```python
from build123d import *

# Parameters (mm, degrees)
F0_R     = 7
F1_DEPTH = 25


with BuildPart() as f1:
    # F0 (on Top) → F1 (new body)
    with BuildSketch(Plane.XY):
        with BuildLine():
            Line((-14, 10.835116), (-14, -7.164884))
            Line((-14, -7.164884), (-7, -14.164884))
            Line((-7, -14.164884), (21.531938, -14.164884))
            ThreePointArc((21.531938, -14.164884), (26.514214, -16.377042), (28.214635, -21.556355))
            ThreePointArc((28.214635, -21.556355), (29.693689, -27.468479), (31.859744, -33.164884))
            Line((31.859744, -33.164884), (38, -33.164884))
            Line((38, -33.164884), (67, -1.89979))
            Line((67, -1.89979), (67, 17.10021))
            Line((67, 17.10021), (62, 22.10021))
            Line((62, 22.10021), (38, 22.10021))
            ThreePointArc((38, 22.10021), (28.531551, 15.73269), (17.158568, 14.809598))
            Line((17.158568, 14.809598), (0, 17.835116))
            Line((0, 17.835116), (-7, 17.835116))
            Line((-7, 17.835116), (-14, 10.835116))
        make_face()
        Circle(F0_R, mode=Mode.SUBTRACT)
    extrude(amount=F1_DEPTH)


solid = f1.part
```
The model under review builds one solid part; all positions refer to its coordinate system, in mm. A direction names the side the tool comes from. Coordinates: 2 decimals unless noted, no trailing zeros. Write each loop counter-clockwise with the first axis right and the second up, starting at its lowest first coordinate (ties: lowest second). Pieces come first, ordered by that corner, then holes. Notation, with made-up numbers: (-12.75, 81) -> (-4.75, 81) arc R27 ccw to (-4.75, 113) -> close; hole circle Ø1 at (-29, -2.5). An arc over 180 degrees is marked (long way). One line per item, written item: value. Start each with the question number.
Q1. To check wall thickness, follow probe 1 along Y at (x, z) = (0, 14.25); probe 2 along X at (y, z) = (0.5, 12.75); probe 3 along Y at (x, z) = (5.5, 18.25). State the ranges of each line that lie inside material, in increasing order.
Q2. For faces 1 (the face through (50, 22.1, 12)), 2 (the face through (8.7, 16.3, 12.3)), 3 (the face through (-3, 17.835, 12)), 4 (the face through (7, -14.165, 12)), list the 3-axis set-ups (+Z, -Z, +X, -X, +Y, -Y) from which the entire face can be reached by the end or side of a thin tool; tool diameter is ignored.
Q3. Add section A-A, the plane y = 0. Give the boundary of the cut face in (x, z), then the cut area to 4 significant figures.
Q4. Add section C-C, the plane z = 10. Give the boundary of the cut face in (x, y).
Q5. Add section B-B, the plane x = 4. Give the boundary of the cut face in (y, z).
Q6. The part is to be moulded in two halves that separate along Y. For faces 5 (the face through (26, 1, 0)), 6 (the face through (6.466, -2.681, 12.325)), 7 (the face through (28.684, 15.787, 12.325)), 8 (the face through (35, -33.165, 12)), say which applies: +Y half, -Y half, draft (parallel to the pull), parting line (faces both ways), or undercut.
Q7. Clearance check with flat-ended pins moving along their axes: P1, Ø12, axis at x = 58.5, z = 16, coming from the -Y side; P2, Ø1, axis at y = -27.5, z = 21, coming from the -X side; P3, Ø1.5, axis at y = 15.5, z = 16, coming from the -X side. State where each tip first meets the part, or that it passes through.
Q8. Add section D-D, the plane y = -26. Give the boundary of the cut face in (x, z).
Response:
1. probe 1: -14.16 to -7, 7 to 17.84
1. probe 2: -14 to -6.98, 6.98 to 67
1. probe 3: -14.16 to -4.33, 4.33 to 16.87
2. face 1: +Z, -Z, +X, -X, +Y
2. face 2: +Z, -Z, +Y
2. face 3: +Z, -Z, -X, +Y
2. face 4: +Z, -Z, -X, -Y
3. outline: (-14, 0) -> (-7, 0) -> (-7, 25) -> (-14, 25) -> close; (7, 0) -> (67, 0) -> (67, 25) -> (7, 25) -> close
3. area: 1,675 mm²
4. outline: (-14, -7.16) -> (-7, -14.16) -> (21.53, -14.16) arc R6.72 cw to (28.21, -21.56) arc R51.58 ccw to (31.86, -33.16) -> (38, -33.16) -> (67, -1.9) -> (67, 17.1) -> (62, 22.1) -> (38, 22.1) arc R22.57 cw to (17.16, 14.81) -> (0, 17.84) -> (-7, 17.84) -> (-14, 10.84) -> close; hole circle Ø14 at (0, 0)
5. outline: (-14.16, 0) -> (-5.74, 0) -> (-5.74, 25) -> (-14.16, 25) -> close; (5.74, 0) -> (17.13, 0) -> (17.13, 25) -> (5.74, 25) -> close
6. face 5: draft
6. face 6: undercut
6. face 7: +Y half
6. face 8: -Y half
7. P1: y = -17.53
7. P2: x = 29.55
7. P3: x = -10.09
8. outline: (29.26, 0) -> (44.65, 0) -> (44.65, 25) -> (29.26, 25) -> close
